Verification items for the finished model (mm, model axes). Round coordinates to 2 decimals unless told otherwise and drop trailing zeros. Order: outer loops, then holes, each group sorted by start corner. A loop starts at its lowest first (then second) coordinate and runs counter-clockwise, first axis right, second up. Notation, with made-up numbers: M -32.75,7.5 L -2.75,7.5 A31 cw -2.75,44.5 Z; hole C -23.5,40 d9. An arc over 180 degrees is marked long. Use CSV: the item, a comma, the result in double quotes. Start each with the question number.
Q1. Sectioned sample at C-C (z = 4.75). Enter the section's corners in (x, y).
Q2. Sectioned sample at B-B (y = 4.5). Enter the section's corners in (x, z).
Q3. Sectioned sample at A-A (x = 13). Enter the section's corners in (y, z), and give its area (3 significant figures).
Q4. Scan lines: line 1 (X direction, y = 20, z = 0.75); line 2 (Y direction, x = 34, z = 2.5). Record each from-to range of solid material in increasing order.
Autodesk Inventor part; units mm, degrees
ref_plane "YZ Plane" through (0, 0, 0) normal (1, 0, 0) x (0, 1, 0)
ref_plane "XZ Plane" through (0, 0, 0) normal (0, 1, 0) x (-1, 0, 0)
ref_plane "XY Plane" through (0, 0, 0) normal (0, 0, 1) x (1, 0, 0)
sketch "Sketch1" plane through (0, 0, 0) normal (0, 0, 1) x (1, 0, 0)
  line L0 (-14.8528, 1.9795) -> (12.8586, 1.9795) construction
  line L1 (12.8586, 1.9795) -> (12.8586, -13.7685) construction
  line L2 (12.8586, -13.7685) -> (-14.8528, -13.7685) construction
  line L3 (-14.8528, -13.7685) -> (-14.8528, 1.9795) construction
  line L4 (5.9975, 1.9795) -> (8.6518, 1.9795) construction
  line L5 (8.6518, 1.9795) -> (8.6518, 4.3671) construction
  line L6 (8.6518, 4.3671) -> (5.9975, 4.3671) construction
  line L7 (5.9975, 4.3671) -> (5.9975, 1.9795) construction
  line L8 (-32.4421, 11.5045) -> (30.2817, 11.5045) construction
  line L9 (-32.4421, 8.3295) -> (29.9988, 8.3295) construction
  line L10 (-13.9321, 13.8921) -> (17.834, 13.8921) construction
  line L11 (-1.8734, -10.8674) -> (-1.8734, -21.0274) construction
  line L12 (-2.2544, -23.9285) -> (-2.2544, -13.7685) construction
  line L13 (-14.8528, -9.4505) -> (-21.958, -9.4505) construction
  line L14 (-21.958, -9.8315) -> (-14.0038, -9.8315) construction
  line L15 (-14.8528, 1.9795) -> (12.6787, 5.1322) construction
  arc A0 (9.1943, 9.241) -> (-14.8528, 1.9795) centre (-1.1526, 0.0577) ccw construction
  circle A1 centre (-10.8004, 5.3198) radius 0.889 construction
  line L16 (-13.0354, 11.5045) -> (-13.0354, 8.3295) construction
  line L17 (10.7302, 11.5045) -> (10.7302, 8.3295) construction
  line L18 (-12.2416, 8.3295) -> (-12.2416, 11.5045) construction
  line L19 (9.9365, 8.3295) -> (9.9365, 11.5045) construction
  line L20 (13.1115, 8.3295) -> (11.9301, 8.1942) construction
  line L21 (11.9301, 8.1942) -> (12.3229, 8.2392) construction
  line L22 (13.377, 6.0111) -> (13.2018, 7.5409) construction
  line L23 (-13.2979, 6.6819) -> (-11.5809, 5.7454) construction
  line L24 (-10.4753, 2.4807) -> (-10.6993, 4.4365) construction
  arc A2 (9.1943, 9.241) -> (11.9301, 8.1942) centre (11.5689, 11.3486) ccw construction
  arc A3 (13.2018, 7.5409) -> (12.3229, 8.2392) centre (12.4132, 7.4506) ccw construction
  arc A4 (12.6787, 5.1322) -> (13.377, 6.0111) centre (12.5884, 5.9208) ccw construction
  circle A5 centre (-11.9953, -0.878) radius 1.5875 construction
  line L25 (-13.5828, 0.7095) -> (-5.6621, 0.7095) construction
  line L26 (-13.5828, -2.3385) -> (-13.5828, 0.7095) construction
  circle A6 centre (10.0011, -10.911) radius 1.5875 construction
  line L27 (11.5886, -9.3235) -> (11.5886, -12.4985) construction
  line L28 (11.5886, -12.4985) -> (4.7585, -12.4985) construction
  line L29 (-13.0354, 11.5045) -> (10.7302, 11.5045) construction
  line L30 (10.7302, 11.5045) -> (10.7302, 21.0295) construction
  line L31 (10.7302, 21.0295) -> (-13.0354, 21.0295) construction
  line L32 (-13.0354, 21.0295) -> (-13.0354, 11.5045) construction
  circle A7 centre (9.2302, 19.5295) radius 1.5 construction
  circle A8 centre (9.2302, 19.5295) radius 30 construction
  circle A9 centre (-11.5354, 13.0045) radius 1.5 construction
  circle A10 centre (-11.5354, 13.0045) radius 30 construction
  line L33 (-41.5354, 49.5295) -> (39.2302, 49.5295)
  line L34 (39.2302, 49.5295) -> (39.2302, -16.9955)
  line L35 (39.2302, -16.9955) -> (-41.5354, -16.9955)
  line L36 (-41.5354, -16.9955) -> (-41.5354, 49.5295)
  line L37 (-105.0354, 113.0295) -> (102.7302, 113.0295)
  line L38 (102.7302, 113.0295) -> (102.7302, -80.4955)
  line L39 (102.7302, -80.4955) -> (-105.0354, -80.4955)
  line L40 (-105.0354, -80.4955) -> (-105.0354, 113.0295)
  point P0 (0, 0)
  dimension "d0" = 27.7114
  dimension "d1" = 15.748
  dimension "d2" = 2.6543
  dimension "buttonHeight" = 2.3876
  dimension "d4" = 3.175
  dimension "d5" = 2.3876
  dimension "buttonInset" = 4.2068
  dimension "d10" = 14.732
  dimension "d11" = 0.381
  dimension "d12" = 10.16
  dimension "d14" = 11.43
  dimension "d15" = 0.381
  dimension "d16" = 6.35
  dimension "nail" = 1.778
  dimension "clearance" = 0.7937
  dimension "d32" = 0.7937
  dimension "cutOutLength" = 23.7656
  dimension "d34" = 2.3813
  dimension "d35" = 1.9558
  dimension "d36" = 1.9558
  dimension "d37" = 3.175
  dimension "d38" = 0.7937
  dimension "holeDistanceFromSurface" = 3.0097
  dimension "holeDistanceFromEnd" = 4.0524
  dimension "d52" = 3.175
  dimension "d53" = 1.27
  dimension "d54" = 1.27
  dimension "d55" = 3.175
  dimension "d56" = 1.27
  dimension "d57" = 1.27
  dimension "d60" = 9.525
  dimension "d69" = 3
  dimension "d70" = 60
  dimension "d71" = 3
  dimension "d72" = 60
  dimension "d75" = 63.5
  dimension "margin" = 63.5
  dimension "d77" = 63.5
  dimension "d78" = 63.5
extrude "Extrusion9" add sketch "Sketch1" along normal blind 6.35
equation "\"d5\" = buttonHeight"
equation "\"d32\" = clearance"
properties part number "Surface Switch Cutout Jig"
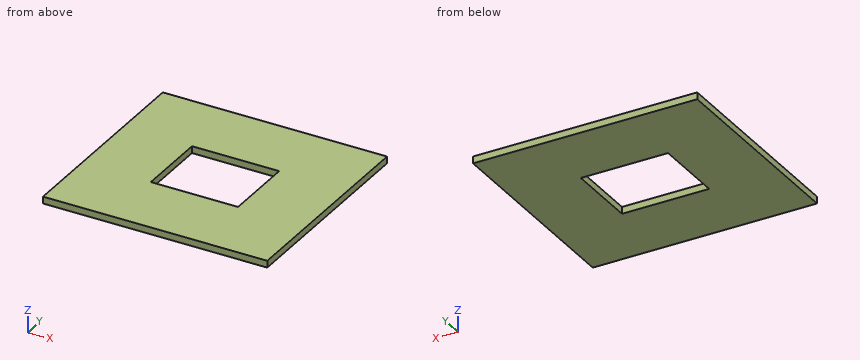
Verdict:
1,outline,"M -105.04,-80.5 L 102.73,-80.5 L 102.73,113.03 L -105.04,113.03 Z; hole M -41.54,-17 L 39.23,-17 L 39.23,49.53 L -41.54,49.53 Z"
2,outline,"M -105.04,0 L -41.54,0 L -41.54,6.35 L -105.04,6.35 Z; M 39.23,0 L 102.73,0 L 102.73,6.35 L 39.23,6.35 Z"
3,outline,"M -80.5,0 L -17,0 L -17,6.35 L -80.5,6.35 Z; M 49.53,0 L 113.03,0 L 113.03,6.35 L 49.53,6.35 Z"
3,area,"806 mm²"
4,line 1,"x = -105.04 to -41.54, 39.23 to 102.73"
4,line 2,"y = -80.5 to -17, 49.53 to 113.03"
